```python
from build123d import *

# Parameters (mm, degrees)
BASE_DEPTH           = 20
SKETCH2_R            = 1.55
CARRIAGESIDE_DEPTH   = 2
SKETCH5_R            = 1.55
CABLECHAINSIDE_DEPTH = 43.355637169
CHAMFER1_SIZE        = 1


with BuildPart() as part:
    # Sketch1 → Base (new body)
    with BuildSketch(Plane.XY):
        Polygon((0, 0), (35, 0), (35, 2), (2, 2), (2, 15), (0, 15), align=None)
    extrude(amount=BASE_DEPTH)

    # Sketch2 → CarriageSide (cut)
    with BuildSketch(Plane.ZY):
        with Locations(Location((14.25, 11, 0), (0, 0, 270))):
            Circle(SKETCH2_R)
        with Locations(Location((5.75, 11, 0), (0, 0, 270))):
            Circle(SKETCH2_R)
    extrude(amount=-CARRIAGESIDE_DEPTH, mode=Mode.SUBTRACT)

    # Sketch5 → CableChainSide (cut, through all)
    with BuildSketch(Plane(origin=(0, 2, 0), x_dir=(1, 0, 0), z_dir=(0, 1, 0))):
        with Locations(Location((21.25, -16, 0), (0, 0, 180))):
            Circle(SKETCH5_R)
        with Locations(Location((28.75, -9.3, 0), (0, 0, 180))):
            Circle(SKETCH5_R)
    extrude(amount=-CABLECHAINSIDE_DEPTH, mode=Mode.SUBTRACT)

    # Chamfer1
    chamfer1_edges = [part.edges().sort_by_distance(p)[0] for p in [
        (35, 1, 20),
        (1, 15, 20),
        (1, 15, 0),
        (35, 1, 0),
    ]]
    chamfer(chamfer1_edges, length=CHAMFER1_SIZE)


solid = part.part
```
Verification items for the finished model (mm, model axes). A direction names the side the tool comes from. Round coordinates to 2 decimals unless told otherwise and drop trailing zeros. Order: outer loops, then holes, each group sorted by start corner. A loop starts at its lowest first (then second) coordinate and runs counter-clockwise, first axis right, second up. Notation, with made-up numbers: (-28, 8.5) -> (-22, 8.5) arc R19 cw to (-22, 13.5) -> close; hole circle Ø3 at (22.5, 37.5). An arc over 180 degrees is marked (long way). Put each result on its own line as item: value. Start each with the question number.
(1) Depth check by flat-ended pin: pin 1 Ø6 at (x, z) = (18.5, 9.5) entering from +Y; pin 2 Ø2 at (y, z) = (12.5, 13) entering from +X. Enter the tip coordinate at first touch or a pass-through.
(2) Section check D-D (z = 3). Enter the section's corners in (x, y).
(3) Section check A-A (z = 9.3). Enter the section's corners in (x, y).
(4) Material ranges on line 1 along Z through (x, y) = (0.95, 11); line 2 along Y through (x, z) = (13.5, 7.75), recorded low to high.
(5) Section check B-B (y = 11). Enter the section's corners in (x, z).
(6) Draft check along Y on faces 3 (the face through (34.5, 1, 0.5)), 4 (the face through (0.99, 12.14, 15.3)), 5 (the face through (1, 15, 10)), 6 (the face through (0.99, 12.55, 5.82)). Enter one of: +Y half, -Y half, draft (parallel to the pull), parting line (faces both ways), or undercut.
(7) Tool access check on faces 1 (the face through (19, 2, 10)), 2 (the face through (17, 0, 10)). Record the directions out of +Z, -Z, +X, -X, +Y, -Y that give a thin tool (end or side, any length) a straight path to the whole face; none if there is none.
(8) Section check C-C (x = 28.75). Enter the section's corners in (y, z).
Completed:
1. pin 1: stops at y = 2
1. pin 2: stops at x = 2
2. outline: (0, 0) -> (35, 0) -> (35, 2) -> (2, 2) -> (2, 15) -> (0, 15) -> close
3. outline: (0, 0) -> (27.2, 0) -> (27.2, 2) -> (2, 2) -> (2, 15) -> (0, 15) -> close; (30.3, 0) -> (35, 0) -> (35, 2) -> (30.3, 2) -> close
4. line 1: z = 0 to 4.2, 7.3 to 12.7, 15.8 to 20
4. line 2: y = 0 to 2
5. outline: (0, 0) -> (2, 0) -> (2, 4.2) -> (0, 4.2) -> close; (0, 7.3) -> (2, 7.3) -> (2, 12.7) -> (0, 12.7) -> close; (0, 15.8) -> (2, 15.8) -> (2, 20) -> (0, 20) -> close
6. face 3: draft
6. face 4: undercut
6. face 5: +Y half
6. face 6: undercut
7. face 1: +Z, -Z, +X, +Y
7. face 2: +Z, -Z, +X, -X, -Y
8. outline: (0, 0) -> (2, 0) -> (2, 7.75) -> (0, 7.75) -> close; (0, 10.85) -> (2, 10.85) -> (2, 20) -> (0, 20) -> close
